Here's how the part is built. I have some questions about the finished solid (model axes, mm). Give positions to 0.01 mm unless a question says otherwise; leave off trailing zeros. Loops run counter-clockwise (first coordinate to the right, second up) from the corner with the lowest first, then second, coordinate; pieces in that order, holes last. Notation, with made-up numbers: (36.25, -36.5) - (51.25, -36.5) arc R17 cw to (51.25, -14.5) - close; hole circle Ø6 at (61, 7.25). An arc over 180 degrees is marked (long way). Return JSON: item names as keys, results as strings. Group by question number.
(1) If we section it at C-C (z = 88): Please give me the cut outline in (x, y), then the cut area to 3 significant figures.
(2) For P1, Ø2, axis at y = -9.5, z = 103.5, coming from the +X side; P2, Ø7.5, axis at x = -41, z = 109.5, coming from the +Y side; P3, Ø1, axis at y = -5, z = 23.5, coming from the -X side, each with a flat end and sliding along its axis, tell me the tip position at first contact or that it passes through.
(3) If we section it at A-A (y = 0.5): Please give me the cut outline in (x, z).
(4) If we section it at B-B (x = 67.5): Please give me the cut outline in (y, z).
(5) I need wall thicknesses on probe 1 along Z at (x, y) = (16, -3); probe 2 along X at (y, z) = (-5.25, 94.5). Which ranges of each line are inside material? Lowest first, please. Write a range as [from, to].
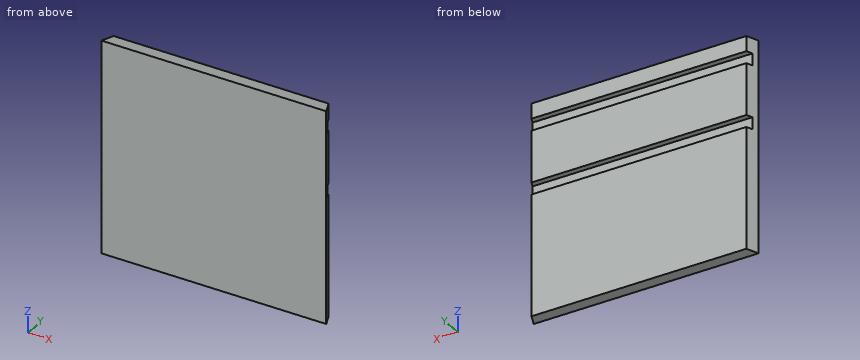
```python
from build123d import *

# Parameters (mm, degrees)
F1_DEPTH = 133.35
F2_W     = 556
F2_H     = 15
F3_DEPTH = 7.5


with BuildPart() as f1:
    # F0 (on Top) → F1 (new body, symmetric)
    with BuildSketch(Plane.XY):
        Polygon((-142.2794159597, -11.8120698132), (128.1365840403, -11.8120698132), (134.3497874759, -11.8120698132), (128.1365840403, 3.1879301868), (108.9945, 3.1879301868), (-30.4355215827, 3.1879301868), (-35.2318651079, 3.1879301868), (-123.1373319193, 3.1879301868), (-142.2794159597, 3.1879301868), (-148.4926193953, -11.8120698132), align=None)
    extrude(amount=F1_DEPTH, both=True)

    # F2 (on face) → F3 (cut)
    with BuildSketch(Plane(origin=(0, 3.1879301868, 0), x_dir=(-1, 0, 0), z_dir=(0, 1, 0))):
        with Locations((5, 26.85)):
            Rectangle(F2_W, F2_H)
        with Locations((5, 106.85)):
            Rectangle(F2_W, F2_H)
    extrude(amount=-F3_DEPTH, mode=Mode.SUBTRACT)


solid = f1.part
```
Values:
{
 "1": {"outline": "(-148.49, -11.81) - (134.35, -11.81) - (128.14, 3.19) - (-142.28, 3.19) - close", "area": "4,150 mm2"},
 "2": {"P1": "x = 133.81", "P2": "y = -4.31", "P3": "x = -145.88"},
 "3": {"outline": "(-143.39, -133.35) - (129.25, -133.35) - (129.25, 19.35) - (-143.39, 19.35) - close; (-143.39, 34.35) - (129.25, 34.35) - (129.25, 99.35) - (-143.39, 99.35) - close; (-143.39, 114.35) - (129.25, 114.35) - (129.25, 133.35) - (-143.39, 133.35) - close"},
 "4": {"outline": "(-11.81, -133.35) - (3.19, -133.35) - (3.19, 19.35) - (-4.31, 19.35) - (-4.31, 34.35) - (3.19, 34.35) - (3.19, 99.35) - (-4.31, 99.35) - (-4.31, 114.35) - (3.19, 114.35) - (3.19, 133.35) - (-11.81, 133.35) - close"},
 "5": {"probe 1": "[-133.35, 19.35], [34.35, 99.35], [114.35, 133.35]", "probe 2": "[-145.77, 131.63]"}
}
